Design review of the part built by this model. Coordinates are the model's own, in mm. A direction names the side the tool comes from. Coordinates: 2 decimals unless noted, no trailing zeros. Write each loop counter-clockwise with the first axis right and the second up, starting at its lowest first coordinate (ties: lowest second). Pieces come first, ordered by that corner, then holes. Notation, with made-up numbers: M -3,13 L 43,13 A7 cw 43,20 Z; hole C 7.25,-0.75 d6. An arc over 180 degrees is marked long. Write item = value, one per line.
```python
from build123d import *

# Parameters (mm, degrees)
SKETCH1_R           = 9.80909091
SKETCH1_R_2         = 3.175
BOSS_EXTRUDE1_DEPTH = 2.794
SKETCH2_R           = 7
SKETCH2_R_2         = 1.1
CUT_EXTRUDE1_DEPTH  = 1.65
SKETCH2_3_R         = 1.1
CUT_EXTRUDE2_DEPTH  = 15.955342623


with BuildPart() as part:
    # Sketch1 → Boss-Extrude1 (new, symmetric)
    with BuildSketch(Plane.XY):
        Circle(SKETCH1_R)
        Circle(SKETCH1_R_2, mode=Mode.SUBTRACT)
    extrude(amount=BOSS_EXTRUDE1_DEPTH, both=True)

    # Sketch2 → Cut-Extrude1 (cut)
    with BuildSketch(Plane.XY.offset(2.794)):
        Circle(SKETCH2_R)
        with Locations((-5.25145, 0)):
            Circle(SKETCH2_R_2, mode=Mode.SUBTRACT)
        with Locations((5.25145, 0)):
            Circle(SKETCH2_R_2, mode=Mode.SUBTRACT)
    cut_extrude1 = extrude(amount=-CUT_EXTRUDE1_DEPTH, mode=Mode.SUBTRACT)

    # Mirror1: Cut-Extrude1 across plane
    add(cut_extrude1.mirror(Plane.XY), mode=Mode.SUBTRACT)

    # Sketch2_3 → Cut-Extrude2 (cut, through all)
    with BuildSketch(Plane.XY.offset(2.794)):
        with BuildLine():
            ThreePointArc((-6.35145, 0), (-5.25145, -1.1), (-4.15145, 0))
            Line((-4.15145, 0), (-6.35145, 0))
        make_face()
        with BuildLine():
            Line((-6.35145, 0), (-4.15145, 0))
            ThreePointArc((-4.15145, 0), (-5.25145, 1.1), (-6.35145, 0))
        make_face()
        with Locations((5.25145, 0)):
            Circle(SKETCH2_3_R)
    extrude(amount=-CUT_EXTRUDE2_DEPTH, mode=Mode.SUBTRACT)


solid = part.part
```
Q1. For P1, Ø4, axis at x = 1.5, y = 3.5, coming from the +Z side; P2, Ø3, axis at y = 2, z = 1, coming from the -X side; P3, Ø3, axis at x = 6.5, z = -1, coming from the +Y side; P4, Ø2, axis at x = -5.25, y = 0, coming from the -Z side, all flat-tipped, find the tip position at first contact; note any pin that passes through.
Check result:
P1 = 1.14
P2 = -9.8
P3 = 8.44
P4 = through
Q2. Consider section C-C, the plane z = 2.35. State the section outline as (x, y) points, and give its area (3 significant figures).
Check result:
outline = C 0,0 d19.62; hole C 0,0 d14
area = 148 mm²
Q3. Wall thickness on line 1 (Y direction, x = 0, z = -0.25) (3 decimals); line 2 (Y direction, x = 0, z = 1.65); line 3 (Z direction, x = -5, y = 2.75): over which ranges is each line inside the solid? List them lowest first.
Check result:
line_1 = -9.809 to -3.175, 3.175 to 9.809
line_2 = -9.81 to -7, 7 to 9.81
line_3 = -1.14 to 1.14
Q4. Machinability: for faces 4 (the cylindrical face through (6.466, -2.681, -1.981)), 5 (the cylindrical face through (-6.35, 0.05, 0.02)), 6 (the flat face through (1.5, -3, 1.144)), which of the approach directions +Z, -Z, +X, -X, +Y, -Y give a long, thin tool a straight path to every point of the face, cutting with its end or side? Answer none if there is none.
Check result:
face_4 = -Z
face_5 = +Z, -Z
face_6 = +Z
Q5. Consider section A-A, the plane x = 0. State the section outline as (y, z) points (3 decimals), and give its area (3 significant figures).
Check result:
outline = M -9.809,-2.794 L -7,-2.794 L -7,-1.144 L -3.175,-1.144 L -3.175,1.144 L -7,1.144 L -7,2.794 L -9.809,2.794 Z; M 3.175,-1.144 L 7,-1.144 L 7,-2.794 L 9.809,-2.794 L 9.809,2.794 L 7,2.794 L 7,1.144 L 3.175,1.144 Z
area = 48.9 mm²
Q6. The part is to be moulded in two halves that separate along Y. For faces 1 (the cylindrical face through (9.356, 2.946, 0.039)), 2 (the flat face through (-7, 2, 2.794)), 3 (the cylindrical face through (6.466, -2.681, 1.981)), say which applies: +Y half, -Y half, draft (parallel to the pull), parting line (faces both ways), or undercut.
Check result:
face_1 = parting line
face_2 = draft
face_3 = undercut
Q7. Consider section D-D, the plane y = 3.75. State the section outline as (x, z) points.
Check result:
outline = M -9.06,-2.79 L -5.91,-2.79 L -5.91,-1.14 L 5.91,-1.14 L 5.91,-2.79 L 9.06,-2.79 L 9.06,2.79 L 5.91,2.79 L 5.91,1.14 L -5.91,1.14 L -5.91,2.79 L -9.06,2.79 Z
Q8. Consider section B-B, the plane y = 0. State the section outline as (x, z) points (3 decimals).
Check result:
outline = M -9.809,-2.794 L -7,-2.794 L -7,-1.144 L -6.351,-1.144 L -6.351,1.144 L -7,1.144 L -7,2.794 L -9.809,2.794 Z; M -4.151,-1.144 L -3.175,-1.144 L -3.175,1.144 L -4.151,1.144 Z; M 3.175,-1.144 L 4.151,-1.144 L 4.151,1.144 L 3.175,1.144 Z; M 6.351,-1.144 L 7,-1.144 L 7,-2.794 L 9.809,-2.794 L 9.809,2.794 L 7,2.794 L 7,1.144 L 6.351,1.144 Z
